For this review, take the finished solid that the model builds, in its own axes (mm). A direction names the side the tool comes from. Coordinates: 2 decimals unless noted, no trailing zeros. Loops run counter-clockwise (first coordinate to the right, second up) from the corner with the lowest first, then second, coordinate; pieces in that order, holes last. Notation, with made-up numbers: M 52.5,24.25 L 75.5,24.25 A12 ccw 75.5,40.25 Z; hole C 59,-39.75 d3. An arc over 180 degrees is marked long. Write item = value, one per line.
from build123d import *

# Parameters (mm, degrees)
PAD_DEPTH = 6


with BuildPart() as part:
    # Sketch → Pad (new body)
    with BuildSketch(Plane.XY):
        with BuildLine():
            ThreePointArc((-4.2, -10.8), (0, -15), (4.2, -10.8))
            Line((4.2, -10.8), (4.2, 0.2))
            ThreePointArc((4.2, 0.2), (0, 4.4), (-4.2, 0.2))
            Line((-4.2, 0.2), (-4.2, -10.8))
        make_face()
        Polygon((-2.35, 0), (-2.35, -1.6), (2.35, -1.6), (2.35, 0), (0.8, 0), (0.8, 3.1), (-0.8, 3.1), (-0.8, 0), align=None, mode=Mode.SUBTRACT)
        with BuildLine():
            ThreePointArc((3, -5.8), (0, -2.8), (-3, -5.8))
            Line((-3, -5.8), (-3, -10.8))
            ThreePointArc((-3, -10.8), (0, -13.8), (3, -10.8))
            Line((3, -10.8), (3, -5.8))
        make_face(mode=Mode.SUBTRACT)
    extrude(amount=PAD_DEPTH)


solid = part.part
Q1. Machinability: for faces 1 (the face through (0, -1.6, 3)), 2 (the face through (-2, -3, 0)), which of the approach directions +Z, -Z, +X, -X, +Y, -Y give a long, thin tool a straight path to every point of the face, cutting with its end or side? Answer none if there is none.
Solved:
face_1 = +Z, -Z
face_2 = -Z, +X, -X, +Y, -Y
Q2. Add section B-B (y = -11.5). Write out the cut boundary in (x, z).
Solved:
outline = M -4.14,0 L -2.92,0 L -2.92,6 L -4.14,6 Z; M 2.92,0 L 4.14,0 L 4.14,6 L 2.92,6 Z
Q3. For pin 1 Ø0.8 at (x, z) = (2, 2.5) entering from -Y; pin 2 Ø1.4 at (x, z) = (1, 3) entering from +Y; pin 3 Ø0.9 at (y, z) = (1, 4) entering from -X, all flat-tipped, find the tip position at first contact; note any pin that passes through.
Solved:
pin_1 = -14.68
pin_2 = 4.39
pin_3 = -4.19
Q4. Add section A-A (x = 0). Write out the cut boundary in (y, z), and give its area (3 significant figures).
Solved:
outline = M -15,0 L -13.8,0 L -13.8,6 L -15,6 Z; M -2.8,0 L -1.6,0 L -1.6,6 L -2.8,6 Z; M 3.1,0 L 4.4,0 L 4.4,6 L 3.1,6 Z
area = 22.2 mm²
Q5. For line 1 along Y through (x, z) = (1.75, 3.1); line 2 along Y through (x, z) = (-1.5, 5.3); line 3 along X through (y, z) = (-0.5, 2.95), list the stretches that pass through material, from the lowest coordinate up.
Solved:
line_1 = -14.62 to -13.24, -3.36 to -1.6, 0 to 4.02
line_2 = -14.72 to -13.4, -3.2 to -1.6, 0 to 4.12
line_3 = -4.2 to -2.35, 2.35 to 4.2
Q6. Add section C-C (z = 4.5). Write out the cut boundary in (x, y), and give its area (3 significant figures).
Solved:
outline = M -4.2,-10.8 A4.2 ccw 4.2,-10.8 L 4.2,0.2 A4.2 ccw -4.2,0.2 Z; hole M -3,-10.8 A3 ccw 3,-10.8 L 3,-5.8 A3 ccw -3,-5.8 Z; hole M -2.35,-1.6 L 2.35,-1.6 L 2.35,0 L 0.8,0 L 0.8,3.1 L -0.8,3.1 L -0.8,0 L -2.35,0 Z
area = 77.1 mm²
Q7. Draft analysis for pull direction X (two halves, no side actions). For faces 3 (the face through (4.2, -5, 3)), 4 (the face through (2, 0, 3)), 5 (the face through (-2, -3, 6)), state which applies: +X half, -X half, draft (parallel to the pull), parting line (faces both ways), or undercut.
Solved:
face_3 = +X half
face_4 = undercut
face_5 = draft
Q8. Add section D-D (x = -1.75). Write out the cut boundary in (y, z).
Solved:
outline = M -14.62,0 L -13.24,0 L -13.24,6 L -14.62,6 Z; M -3.36,0 L -1.6,0 L -1.6,6 L -3.36,6 Z; M 0,0 L 4.02,0 L 4.02,6 L 0,6 Z
